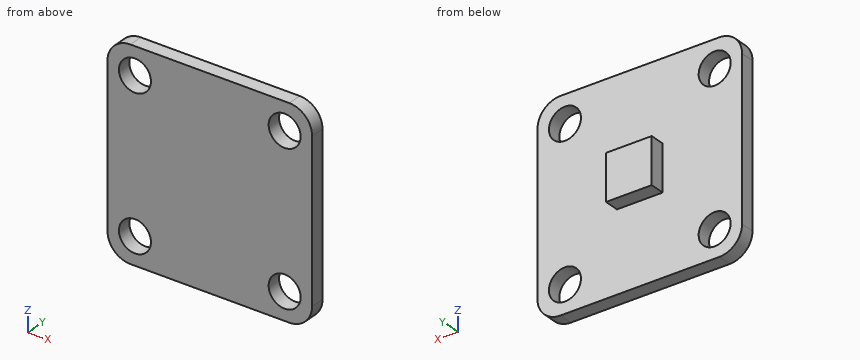
from build123d import *

# Parameters (mm, degrees)
SKETCH1_W           = 22.733
SKETCH1_H           = 22.733
BOSS_EXTRUDE1_DEPTH = 1.5748
FILLET1_R           = 2.54
SKETCH2_R           = 1.778
CUT_EXTRUDE1_DEPTH  = 1.5748
SKETCH3_W           = 5.08
SKETCH3_H           = 5.08
BOSS_EXTRUDE2_DEPTH = 1.651


with BuildPart() as part:
    # Sketch1 → Boss-Extrude1 (new body)
    with BuildSketch(Plane.XZ.offset(-26.884)):
        with Locations((11.43, 0)):
            Rectangle(SKETCH1_W, SKETCH1_H)
    extrude(amount=BOSS_EXTRUDE1_DEPTH)

    # Fillet1
    fillet1_edges = [part.edges().sort_by_distance(p)[0] for p in [
        (0.0635, 26.0966, 11.3665),
        (22.7965, 26.0966, 11.3665),
        (22.7965, 26.0966, -11.3665),
        (0.0635, 26.0966, -11.3665),
    ]]
    fillet(fillet1_edges, radius=FILLET1_R)

    # Sketch2 → Cut-Extrude1 (cut)
    with BuildSketch(Plane(origin=(0, 26.884, 0), x_dir=(1, 0, 0), z_dir=(0, 1, 0))):
        with Locations(Location((19.7485, 8.3185, 0), (0, 0, 270))):
            Circle(SKETCH2_R)
        with Locations(Location((3.1115, 8.3185, 0), (0, 0, 90))):
            Circle(SKETCH2_R)
        with Locations(Location((19.7485, -8.3185, 0), (0, 0, 90))):
            Circle(SKETCH2_R)
        with Locations(Location((3.1115, -8.3185, 0), (0, 0, 270))):
            Circle(SKETCH2_R)
    extrude(amount=-CUT_EXTRUDE1_DEPTH, mode=Mode.SUBTRACT)

    # Sketch3 → Boss-Extrude2 (add)
    with BuildSketch(Plane(origin=(0, 26.884, 0), x_dir=(1, 0, 0), z_dir=(0, 1, 0))):
        with Locations((11.43, 0)):
            Rectangle(SKETCH3_W, SKETCH3_H)
    extrude(amount=BOSS_EXTRUDE2_DEPTH)


solid = part.part
Source: CAD feature listing. Evaluate the final solid. Frame: model axes, mm. Coordinates: 2 decimals unless noted, no trailing zeros. Loops run counter-clockwise (first coordinate to the right, second up) from the corner with the lowest first, then second, coordinate; pieces in that order, holes last. Notation, with made-up numbers: (11.25, 21) - (20.25, 21) arc R13 ccw to (20.25, 38) - close; hole circle Ø10 at (21, 60). An arc over 180 degrees is marked (long way). Return JSON: item names as keys, results as strings.
Q1. Section D-D, the plane z = -3.25. Return loops of the section in (x, y), plus the area to 3 significant figures.
Results:
{"outline": "(0.06, 25.31) - (22.8, 25.31) - (22.8, 26.88) - (0.06, 26.88) - close", "area": "35.8 mm2"}
Q2. Material intervals for line 1 along X through (y, z) = (25.75, 9.75); line 2 along Z through (x, y) = (13.25, 28.05); line 3 along Y through (x, z) = (15.5, 0.25), sorted ascending.
Results:
{"line 1": "0.24 to 2.06, 4.17 to 18.69, 20.8 to 22.62", "line 2": "-2.54 to 2.54", "line 3": "25.31 to 26.88"}
Q3. Section A-A, the plane x = 4.5. Return loops of the section in (y, z), plus the area to 3 significant figures.
Results:
{"outline": "(25.31, -11.37) - (26.88, -11.37) - (26.88, -9.43) - (25.31, -9.43) - close; (25.31, -7.21) - (26.88, -7.21) - (26.88, 7.21) - (25.31, 7.21) - close; (25.31, 9.43) - (26.88, 9.43) - (26.88, 11.37) - (25.31, 11.37) - close", "area": "28.8 mm2"}
Q4. Section C-C, the plane x = 12. Return loops of the section in (y, z) (1 decimal).
Results:
{"outline": "(25.3, -11.4) - (26.9, -11.4) - (26.9, -2.5) - (28.5, -2.5) - (28.5, 2.5) - (26.9, 2.5) - (26.9, 11.4) - (25.3, 11.4) - close"}
Q5. Section B-B, the plane y = 25.6. Return loops of the section in (x, z).
Results:
{"outline": "(0.06, -8.83) arc R2.54 ccw to (2.6, -11.37) - (20.26, -11.37) arc R2.54 ccw to (22.8, -8.83) - (22.8, 8.83) arc R2.54 ccw to (20.26, 11.37) - (2.6, 11.37) arc R2.54 ccw to (0.06, 8.83) - close; hole circle Ø3.56 at (3.11, -8.32); hole circle Ø3.56 at (3.11, 8.32); hole circle Ø3.56 at (19.75, -8.32); hole circle Ø3.56 at (19.75, 8.32)"}
Q6. Contact query for flat-ended pins moving along their axis: P1, Ø1.8, axis at y = 27.5, z = -1, coming from the +X side; P2, Ø3, axis at x = 3.11, z = -8.32, coming from the +Y side; P3, Ø1.8, axis at y = 28, z = -0.5, coming from the -X side; P4, Ø1, axis at x = 16, z = 4.5, coming from the +Y side. Output: stop coordinate, or through.
Results:
{"P1": "x = 22.8", "P2": "through", "P3": "x = 8.89", "P4": "y = 26.88"}
